```python
from build123d import *

# Parameters (mm, degrees)
EXTRUDE1_DEPTH     = 30
FILLET1_R          = 2.54
CUT_EXTRUDE1_REACH = 71.778
SKETCH2_R          = 2.5
CUT_EXTRUDE2_REACH = 71.778
SKETCH3_W          = 3.948997199
SKETCH3_H          = 2.915862496
SKETCH3_W_2        = 5.260004778
SKETCH3_W_3        = 4.51085759
EXTRUDE2_DEPTH     = 7.004916842
SKETCH5_R          = 11.43
EXTRUDE3_DEPTH     = 3.175
FILLET2_R          = 2.54
FILLET3_R          = 1.27
SKETCH6_R          = 3.013004542
EXTRUDE4_DEPTH     = 8.025


with BuildPart() as part:
    # Sketch1 → Extrude1 (new body)
    with BuildSketch(Plane.XY):
        Polygon((-33.5, 17.102458421), (-41.5, 17.102458421), (-41.5, 22.102458421), (-33.5, 22.102458421), (-33.5, 25.297541579), (-10.877689124, 25.297541579), (-10.877689124, 32.302458421), (33.5, 32.302458421), (33.5, 22.102458421), (41.5, 22.102458421), (41.5, 17.102458421), (33.5, 17.102458421), (33.5, -25.297541579), (-33.5, -25.297541579), align=None)
    extrude(amount=EXTRUDE1_DEPTH)

    # Fillet1
    fillet1_edges = [part.edges().sort_by_distance(p)[0] for p in [
        (33.5, -4.097541579, 30),
        (-41.5, 19.602458421, 0),
        (41.5, 19.602458421, 30),
        (41.5, 19.602458421, 0),
        (33.5, -4.097541579, 0),
        (0, -25.297541579, 0),
        (-33.5, -4.097541579, 0),
        (33.5, -25.297541579, 15),
        (-33.5, -25.297541579, 15),
        (-33.5, -4.097541579, 30),
        (-41.5, 19.602458421, 30),
        (0, -25.297541579, 30),
    ]]
    fillet(fillet1_edges, radius=FILLET1_R)

    # Sketch2 → Cut-Extrude1 (cut, up to next)
    with BuildSketch(Plane(origin=(0, 22.102458421, 0), x_dir=(1, 0, 0), z_dir=(0, 1, 0)), mode=Mode.PRIVATE) as cut_extrude1_sk1:
        with Locations(Location((-37.5, -6, 0), (0, 0, 270))):
            Circle(SKETCH2_R)
    cut_extrude1_tool1 = extrude(cut_extrude1_sk1.sketch, amount=-CUT_EXTRUDE1_REACH, mode=Mode.PRIVATE) & part.part
    # Sketch2 → Cut-Extrude1 (cut, up to next)
    with BuildSketch(Plane(origin=(0, 22.102458421, 0), x_dir=(1, 0, 0), z_dir=(0, 1, 0)), mode=Mode.PRIVATE) as cut_extrude1_sk2:
        with Locations(Location((-37.5, -24, 0), (0, 0, 270))):
            Circle(SKETCH2_R)
    cut_extrude1_tool2 = extrude(cut_extrude1_sk2.sketch, amount=-CUT_EXTRUDE1_REACH, mode=Mode.PRIVATE) & part.part
    # Sketch2 → Cut-Extrude1 (cut, up to next)
    with BuildSketch(Plane(origin=(0, 22.102458421, 0), x_dir=(1, 0, 0), z_dir=(0, 1, 0)), mode=Mode.PRIVATE) as cut_extrude1_sk3:
        with Locations(Location((37.5, -6, 0), (0, 0, 270))):
            Circle(SKETCH2_R)
    cut_extrude1_tool3 = extrude(cut_extrude1_sk3.sketch, amount=-CUT_EXTRUDE1_REACH, mode=Mode.PRIVATE) & part.part
    # Sketch2 → Cut-Extrude1 (cut, up to next)
    with BuildSketch(Plane(origin=(0, 22.102458421, 0), x_dir=(1, 0, 0), z_dir=(0, 1, 0)), mode=Mode.PRIVATE) as cut_extrude1_sk4:
        with Locations(Location((37.5, -24, 0), (0, 0, 270))):
            Circle(SKETCH2_R)
    cut_extrude1_tool4 = extrude(cut_extrude1_sk4.sketch, amount=-CUT_EXTRUDE1_REACH, mode=Mode.PRIVATE) & part.part
    add(cut_extrude1_tool1.solids().sort_by_distance((-37.5, 22.102458, 6))[0], mode=Mode.SUBTRACT)
    add(cut_extrude1_tool2.solids().sort_by_distance((-37.5, 22.102458, 24))[0], mode=Mode.SUBTRACT)
    add(cut_extrude1_tool3.solids().sort_by_distance((37.5, 22.102458, 6))[0], mode=Mode.SUBTRACT)
    add(cut_extrude1_tool4.solids().sort_by_distance((37.5, 22.102458, 24))[0], mode=Mode.SUBTRACT)

    # Sketch3 → Cut-Extrude2 (cut, up to next)
    with BuildSketch(Plane(origin=(0, 22.102458421, 0), x_dir=(1, 0, 0), z_dir=(0, 1, 0)), mode=Mode.PRIVATE) as cut_extrude2_sk1:
        with Locations((-39.525501401, -6)):
            Rectangle(SKETCH3_W, SKETCH3_H)
    cut_extrude2_tool1 = extrude(cut_extrude2_sk1.sketch, amount=-CUT_EXTRUDE2_REACH, mode=Mode.PRIVATE) & part.part
    # Sketch3 → Cut-Extrude2 (cut, up to next)
    with BuildSketch(Plane(origin=(0, 22.102458421, 0), x_dir=(1, 0, 0), z_dir=(0, 1, 0)), mode=Mode.PRIVATE) as cut_extrude2_sk2:
        with Locations((-39.525501401, -24)):
            Rectangle(SKETCH3_W, SKETCH3_H)
    cut_extrude2_tool2 = extrude(cut_extrude2_sk2.sketch, amount=-CUT_EXTRUDE2_REACH, mode=Mode.PRIVATE) & part.part
    # Sketch3 → Cut-Extrude2 (cut, up to next)
    with BuildSketch(Plane(origin=(0, 22.102458421, 0), x_dir=(1, 0, 0), z_dir=(0, 1, 0)), mode=Mode.PRIVATE) as cut_extrude2_sk3:
        with Locations((38.869997611, -6)):
            Rectangle(SKETCH3_W_2, SKETCH3_H)
    cut_extrude2_tool3 = extrude(cut_extrude2_sk3.sketch, amount=-CUT_EXTRUDE2_REACH, mode=Mode.PRIVATE) & part.part
    # Sketch3 → Cut-Extrude2 (cut, up to next)
    with BuildSketch(Plane(origin=(0, 22.102458421, 0), x_dir=(1, 0, 0), z_dir=(0, 1, 0)), mode=Mode.PRIVATE) as cut_extrude2_sk4:
        with Locations((39.244571205, -24)):
            Rectangle(SKETCH3_W_3, SKETCH3_H)
    cut_extrude2_tool4 = extrude(cut_extrude2_sk4.sketch, amount=-CUT_EXTRUDE2_REACH, mode=Mode.PRIVATE) & part.part
    add(cut_extrude2_tool1.solids().sort_by_distance((-39.525501, 22.102458, 6))[0], mode=Mode.SUBTRACT)
    add(cut_extrude2_tool2.solids().sort_by_distance((-39.525501, 22.102458, 24))[0], mode=Mode.SUBTRACT)
    add(cut_extrude2_tool3.solids().sort_by_distance((38.869998, 22.102458, 6))[0], mode=Mode.SUBTRACT)
    add(cut_extrude2_tool4.solids().sort_by_distance((39.244571, 22.102458, 24))[0], mode=Mode.SUBTRACT)

    # Sketch4 → Extrude2 (add)
    with BuildSketch(Plane(origin=(0, 25.297541579, 0), x_dir=(1, 0, 0), z_dir=(0, 1, 0))):
        with BuildLine():
            Line((-10.877689124, -5.869768646), (-10.877689124, -24.130231354))
            ThreePointArc((-10.877689124, -24.130231354), (-20.007920479, -15), (-10.877689124, -5.869768646))
        make_face()
    extrude(amount=EXTRUDE2_DEPTH)

    # Sketch5 → Extrude3 (add)
    with BuildSketch(Plane(origin=(0, 32.302458421, 0), x_dir=(1, 0, 0), z_dir=(0, 1, 0))):
        with Locations(Location((18.5, -15, 0), (0, 0, 90))):
            Circle(SKETCH5_R)
    extrude(amount=EXTRUDE3_DEPTH)

    # Fillet2
    fillet2_edges = [part.edges().sort_by_distance(p)[0] for p in [
        (18.5, 35.477458421, 26.43),
    ]]
    fillet(fillet2_edges, radius=FILLET2_R)

    # Fillet3
    fillet3_edges = [part.edges().sort_by_distance(p)[0] for p in [
        (-20.007920479, 32.302458421, 15),
    ]]
    fillet(fillet3_edges, radius=FILLET3_R)

    # Sketch6 → Extrude4 (add)
    with BuildSketch(Plane(origin=(0, 35.477458421, 0), x_dir=(1, 0, 0), z_dir=(0, 1, 0))):
        with Locations(Location((18.5, -15, 0), (0, 0, 180))):
            Circle(SKETCH6_R)
    extrude(amount=EXTRUDE4_DEPTH)


solid = part.part
```
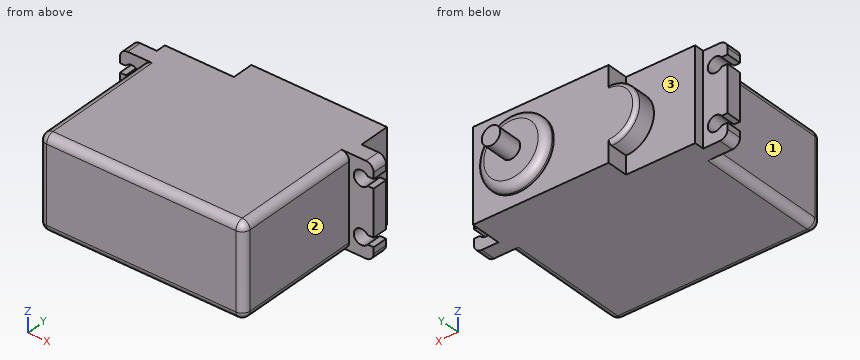
Here's how the part is built. I have some questions about the finished solid (model axes, mm). Face numbers are marked on the shaded views. A direction names the side the tool comes from. Give positions to 0.01 mm unless a question says otherwise; leave off trailing zeros. Order: outer loops, then holes, each group sorted by start corner. A loop starts at its lowest first (then second) coordinate and runs counter-clockwise, first axis right, second up. Notation, with made-up numbers: (-30, 68.25) -> (-23, 68.25) arc R27 ccw to (-23, 87.25) -> close; hole circle Ø9 at (45, 21). An arc over 180 degrees is marked (long way). Use CSV: the item, a comma, the result in double quotes. Start each with the question number.
Item 1: Suppose I cut it at C-C (z = 15). List the corners of the cut face in (x, y) for me.
Item 2: Suppose I cut it at A-A (y = -5.5). List the corners of the cut face in (x, z) for me.
Item 3: Suppose I cut it at D-D (y = 23.5). List the corners of the cut face in (x, z) for me.
Item 4: Suppose I cut it at B-B (x = 18.5). List the corners of the cut face in (y, z) for me, and give its area (3 significant figures).
Item 5: I'm going to push flat-ended pins straight in: P1, Ø1.6, axis at x = 40, y = 20.5, coming from the -Z side; P2, Ø6.5, axis at x = 37.5, z = 6, coming from the -Y side; P3, Ø10, axis at y = 6.5, z = 21, coming from the +X side. Where does each tip first touch, or does it pass through?
Item 6: On a 3-axis mill with a long thin cutter (end or side, diameter ignored), from which of +Z, -Z, +X, -X, +Y, -Y can I reach the whole of each face in a straight line? I mean the marked faces 1, 2 and 3. Say none if no direction works.
Item 7: If I drill on probe 1 along Z at (x, y) = (-37.5, 20.95); probe 2 along Z at (x, y) = (-37, 20); probe 3 along Y at (x, z) = (-15, 4.5), over which ranges is the centre line in solid material (lowest first)? Write a range as [from, to].
Answer block:
1,outline,"(-41.5, 17.1) -> (-33.5, 17.1) -> (-33.5, -22.76) arc R2.54 ccw to (-30.96, -25.3) -> (30.96, -25.3) arc R2.54 ccw to (33.5, -22.76) -> (33.5, 17.1) -> (41.5, 17.1) -> (41.5, 22.1) -> (33.5, 22.1) -> (33.5, 32.3) -> (29.93, 32.3) -> (29.93, 32.94) arc R2.54 ccw to (27.39, 35.48) -> (21.51, 35.48) -> (21.51, 43.5) -> (15.49, 43.5) -> (15.49, 35.48) -> (9.61, 35.48) arc R2.54 ccw to (7.07, 32.94) -> (7.07, 32.3) -> (-18.74, 32.3) arc R1.27 ccw to (-20.01, 31.03) -> (-20.01, 25.3) -> (-33.5, 25.3) -> (-33.5, 22.1) -> (-41.5, 22.1) -> close"
2,outline,"(-33.5, 2.54) arc R2.54 ccw to (-30.96, 0) -> (30.96, 0) arc R2.54 ccw to (33.5, 2.54) -> (33.5, 27.46) arc R2.54 ccw to (30.96, 30) -> (-30.96, 30) arc R2.54 ccw to (-33.5, 27.46) -> close"
3,outline,"(-33.5, 0) -> (33.5, 0) -> (33.5, 30) -> (-33.5, 30) -> close"
4,outline,"(-25.3, 2.54) arc R2.54 ccw to (-22.76, 0) -> (32.3, 0) -> (32.3, 3.57) -> (32.94, 3.57) arc R2.54 ccw to (35.48, 6.11) -> (35.48, 11.99) -> (43.5, 11.99) -> (43.5, 18.01) -> (35.48, 18.01) -> (35.48, 23.89) arc R2.54 ccw to (32.94, 26.43) -> (32.3, 26.43) -> (32.3, 30) -> (-22.76, 30) arc R2.54 ccw to (-25.3, 27.46) -> close"
4,area,"1,840 mm^2"
5,P1,"stops at z = 0.01"
5,P2,"stops at y = 17.1"
5,P3,"stops at x = 33.5"
6,face 1,"+Z, -Z, -X, -Y"
6,face 2,"+Z, -Z, +X, -Y"
6,face 3,"-X, +Y"
7,probe 1,"z = [0, 3.5], [8.5, 21.5], [26.5, 30]"
7,probe 2,"z = [0, 3.55], [8.45, 21.55], [26.45, 30]"
7,probe 3,"y = [-25.3, 25.3]"
